Source: CAD feature listing. Evaluate the final solid. Frame: model axes, mm. Round coordinates to 2 decimals unless told otherwise and drop trailing zeros. Loops run counter-clockwise (first coordinate to the right, second up) from the corner with the lowest first, then second, coordinate; pieces in that order, holes last. Notation, with made-up numbers: M -5.75,46 L 51.25,46 A20 ccw 51.25,69 Z; hole C 81,72.25 d9. An arc over 180 degrees is marked long. Answer as CSV lines item,"result". Start each with the question number.
```python
from build123d import *

# Parameters (mm, degrees)
SKETCH1_R           = 25.5
BOSS_EXTRUDE1_DEPTH = 1.5
SKETCH2_R           = 26
BOSS_EXTRUDE2_DEPTH = 0.75
SKETCH3_R           = 0.6
CUT_EXTRUDE1_DEPTH  = 1.75


with BuildPart() as part:
    # Sketch1 → Boss-Extrude1 (new body)
    with BuildSketch(Plane(origin=(0, 0, 0), x_dir=(1, 0, 0), z_dir=(0, 1, 0))):
        Circle(SKETCH1_R)
    extrude(amount=-BOSS_EXTRUDE1_DEPTH)

    # Sketch2 → Boss-Extrude2 (add)
    with BuildSketch(Plane(origin=(0, -1.5, 0), x_dir=(-1, 0, 0), z_dir=(0, -1, 0))):
        Circle(SKETCH2_R)
    extrude(amount=-BOSS_EXTRUDE2_DEPTH)

    # Sketch3 → Cut-Extrude1 (cut, through all)
    with BuildSketch(Plane(origin=(0, -0.75, 0), x_dir=(1, 0, 0), z_dir=(0, 1, 0))):
        Circle(SKETCH3_R)
    extrude(amount=-CUT_EXTRUDE1_DEPTH, mode=Mode.SUBTRACT)

    # Sketch4 → Cut-Revolve1 (revolve, cut)
    with BuildSketch(Plane.XY):
        Polygon((-4.35, -1.5), (0, -1.5), (0, 0), (-0.55, 0), (-0.55, -0.2), align=None)
    revolve(axis=Axis((0, -1.5, 0), (0, 1, 0)), mode=Mode.SUBTRACT)


solid = part.part
```
1) Section B-B, the plane z = -21. Return loops of the section in (x, y).
2) Section C-C, the plane y = -1.05. Return loops of the section in (x, z), and give its area (3 significant figures).
3) Section A-A, the plane x = -20.5. Return loops of the section in (y, z).
4) Contact query for a flat-ended pin moving along its axis: pin 1 Ø1.4 at (x, z) = (0, 0) entering from -Y. Output: stop coordinate, or through.
5) Ray query, line 1 along Z through (x, y) = (0, -0.1); line 2 along X through (y, z) = (-0.6, 21.5); line 3 along Z through (x, y) = (-6.5, -0.6). Return the intervals inside material, ascending.
6) Mould query, pull axis X, two halves, no side actions, for faces 1 (the conical face through (-0.36, -0.28, -0.7)), 2 (the cylindrical face through (-5.5, -0.4, 24.9)), 3 (the flat face through (-19.1, -0.75, 17.2)). Classes: pulls with the +X half, pulls with the -X half, needs draft (parallel to the pull), parting line crosses it, or undercut.
Findings below:
1,outline,"M -15.33,-1.5 L 15.33,-1.5 L 15.33,-0.75 L 14.47,-0.75 L 14.47,0 L -14.47,0 L -14.47,-0.75 L -15.33,-0.75 Z"
2,outline,"C 0,0 d52; hole C 0,0 d6.07"
2,area,"2,090 mm²"
3,outline,"M -1.5,-15.99 L -0.75,-15.99 L -0.75,-15.17 L 0,-15.17 L 0,15.17 L -0.75,15.17 L -0.75,15.99 L -1.5,15.99 Z"
4,pin 1,"y = -0.25"
5,line 1,"-25.5 to -0.55, 0.55 to 25.5"
5,line 2,"-13.71 to 13.71"
5,line 3,"-24.66 to 24.66"
6,face 1,"undercut"
6,face 2,"parting line crosses it"
6,face 3,"needs draft"
